Could you check a few things on this drawing? It's one solid part, dimensions in mm from its lowest x, y, z. A direction names the side the tool comes from. Give positions to 0.01 mm unless a question says otherwise; leave off trailing zeros. Order: outer loops, then holes, each group sorted by start corner. A loop starts at its lowest first (then second) coordinate and runs counter-clockwise, first axis right, second up.
Item 1: I want a section at A-A, the plane z = 10. Write out the boundary of the cut face in (x, y).
Item 2: I want a section at C-C, the plane y = 6.35. Write out the boundary of the cut face in (x, z).
Item 3: I want a section at D-D, the plane x = 32. Write out the boundary of the cut face in (y, z), then the cut area to 3 significant figures.
Item 4: I'm going to push flat-ended pins straight in: pin 1 Ø5 at (x, y) = (4, 5.5) entering from -Z; pin 2 Ø5 at (y, z) = (10, 4) entering from -X; pin 3 Ø1.5 at (x, y) = (65.5, 8.5) entering from +Z. Where does each tip first touch, or does it pass through?
Item 5: If we mould it in two halves opening along X, with no side actions, what happens to the marked faces 3, 4 and 5? For each: +X half, -X half, draft (parallel to the pull), parting line (faces both ways), or undercut.
Item 6: I want a section at B-B, the plane x = 140.97. Write out the boundary of the cut face in (y, z).
Item 7: Which directions (+Z, -Z, +X, -X, +Y, -Y) give clear straight access to the entire face, cutting with the end or side of a thin tool? Please do the marked faces 1 and 2.
Item 8: If I drill on line 1 along Y through (x, z) = (140.97, 32.7); line 2 along X through (y, z) = (0.75, 9.5); line 3 along X through (y, z) = (6, 32), over which ranges is the centre line in solid material (lowest first)?
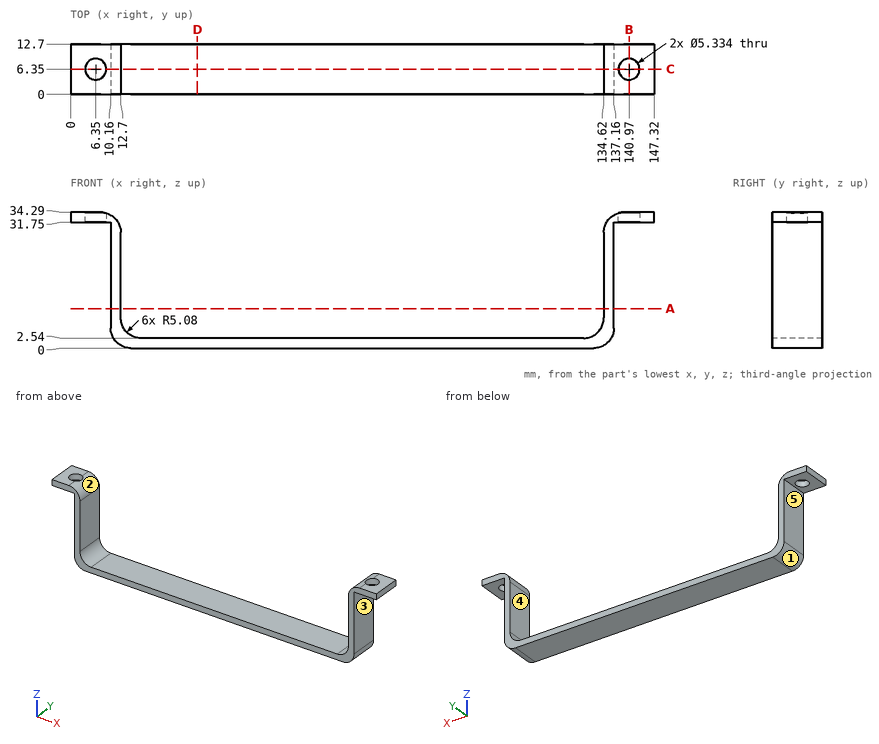
Results list:
1. outline: (10.16, 0) - (12.7, 0) - (12.7, 12.7) - (10.16, 12.7) - close; (134.62, 0) - (137.16, 0) - (137.16, 12.7) - (134.62, 12.7) - close
2. outline: (0, 31.75) - (3.68, 31.75) - (3.68, 34.29) - (0, 34.29) - close; (9.02, 31.75) - (10.16, 31.75) - (10.16, 5.08) arc R5.08 ccw to (15.24, 0) - (132.08, 0) arc R5.08 ccw to (137.16, 5.08) - (137.16, 31.75) - (138.3, 31.75) - (138.3, 34.09) arc R5.08 ccw to (134.62, 29.21) - (134.62, 7.62) arc R5.08 cw to (129.54, 2.54) - (17.78, 2.54) arc R5.08 cw to (12.7, 7.62) - (12.7, 29.21) arc R5.08 ccw to (9.02, 34.09) - close; (143.64, 31.75) - (147.32, 31.75) - (147.32, 34.29) - (143.64, 34.29) - close
3. outline: (0, 0) - (12.7, 0) - (12.7, 2.54) - (0, 2.54) - close
3. area: 32.3 mm2
4. pin 1: stops at z = 31.75
4. pin 2: stops at x = 10.16
4. pin 3: stops at z = 2.54
5. face 3: +X half
5. face 4: undercut
5. face 5: -X half
6. outline: (0, 31.75) - (3.68, 31.75) - (3.68, 34.29) - (0, 34.29) - close; (9.02, 31.75) - (12.7, 31.75) - (12.7, 34.29) - (9.02, 34.29) - close
7. face 1: -Z, -X, +Y, -Y
7. face 2: +Z, +Y, -Y
8. line 1: y = 0 to 3.68, 9.02 to 12.7
8. line 2: x = 10.16 to 12.7, 134.62 to 137.16
8. line 3: x = 0 to 3.71, 8.99 to 11.87, 135.45 to 138.33, 143.61 to 147.32
